```python
from build123d import *

# Parameters (mm, degrees)
SKETCH_1_R               = 32
EXTRUDE_1_DEPTH          = 10
EXTRUDE_2_DEPTH          = 10
PATTERN_CIRCULAR_1_COUNT = 3
SKETCH_3_R               = 23
EXTRUDE_3_DEPTH          = 28
SKETCH_4_R               = 15
CUT_EXTRUDE_1_DEPTH      = 88.68422222
SKETCH_5_R               = 19
CUT_EXTRUDE_2_DEPTH      = 9
SKETCH_6_R               = 4.5
CUT_EXTRUDE_3_DEPTH      = 84.836285858


with BuildPart() as part:
    # Sketch 1 → Extrude 1 (new body)
    with BuildSketch(Plane.XY):
        Circle(SKETCH_1_R)
    extrude(amount=EXTRUDE_1_DEPTH)

    # Sketch 2 → Extrude 2 (add)
    with BuildSketch(Plane.XY):
        with BuildLine():
            Line((20, -11), (48, -11))
            ThreePointArc((48, -11), (59, 0), (48, 11))
            Line((48, 11), (20, 11))
            ThreePointArc((20, 11), (9, 0), (20, -11))
        make_face()
    extrude_2 = extrude(amount=EXTRUDE_2_DEPTH)

    # Pattern Circular 1: Extrude 2 ×3 about axis
    pattern_circular_1_axis = Axis((0, 0, 0), (0, 0, 1))
    for i in range(1, PATTERN_CIRCULAR_1_COUNT):
        add(extrude_2.rotate(pattern_circular_1_axis, i * 360 / PATTERN_CIRCULAR_1_COUNT))

    # Sketch 3 → Extrude 3 (add)
    with BuildSketch(Plane.XY.offset(10)):
        Circle(SKETCH_3_R)
    extrude(amount=EXTRUDE_3_DEPTH)

    # Sketch 4 → Cut-Extrude 1 (cut, through all)
    with BuildSketch(Plane.XY.offset(38)):
        Circle(SKETCH_4_R)
    extrude(amount=-CUT_EXTRUDE_1_DEPTH, mode=Mode.SUBTRACT)

    # Sketch 5 → Cut-Extrude 2 (cut)
    with BuildSketch(Plane.XY.offset(38)):
        Circle(SKETCH_5_R)
    extrude(amount=-CUT_EXTRUDE_2_DEPTH, mode=Mode.SUBTRACT)

    # Sketch 6 → Cut-Extrude 3 (cut, through all)
    with BuildSketch(Plane.XY.offset(10)):
        with Locations((48, 0)):
            Circle(SKETCH_6_R)
        with Locations((-24, 41.569219)):
            Circle(SKETCH_6_R)
        with Locations((-24, -41.569219)):
            Circle(SKETCH_6_R)
    extrude(amount=-CUT_EXTRUDE_3_DEPTH, mode=Mode.SUBTRACT)


solid = part.part
```
Read the model definition and answer for the solid it produces. Units are mm, in the model's axes. A direction names the side the tool comes from. Give positions to 0.01 mm unless a question says otherwise; leave off trailing zeros. Order: outer loops, then holes, each group sorted by start corner. A loop starts at its lowest first (then second) coordinate and runs counter-clockwise, first axis right, second up. Notation, with made-up numbers: (65, 59) -> (99, 59) arc R13 cw to (99, 65) -> close; hole circle Ø7 at (58, 62.5). An arc over 180 degrees is marked (long way). Write item = value, one per line.
1. A cutting plane is placed at D-D, the plane y = -12.5. Write down the section's boundary in (x, z).
Numbers:
outline = (-29.46, 0) -> (-8.29, 0) -> (-8.29, 29) -> (-14.31, 29) -> (-14.31, 38) -> (-19.31, 38) -> (-19.31, 10) -> (-29.46, 10) -> close; (8.29, 0) -> (29.46, 0) -> (29.46, 10) -> (19.31, 10) -> (19.31, 38) -> (14.31, 38) -> (14.31, 29) -> (8.29, 29) -> close
2. Straight lines are drawn through the part: line 1 along X through (y, z) = (-3.5, 2.5); line 2 along Y through (x, z) = (0, 36); line 3 along Z through (x, y) = (-0.5, 15.5). For each, find the intervals that lie inside material, in ascending order.
Numbers:
line_1 = -31.81 to -14.59, 14.59 to 45.17, 50.83 to 58.43
line_2 = -23 to -19, 19 to 23
line_3 = 0 to 29
3. For faces 1 (the face through (-11, -21, 10)), 2 (the face through (-29.1, 28.4, 4.9)), 3 (the face through (39, -11, 5)), determine the directions among +Z, -Z, +X, -X, +Y, -Y from which every point of the face is accessible in a straight line to the end or side of a thin tool.
Numbers:
face_1 = +Z
face_2 = +Z, -Z, -X
face_3 = +Z, -Z, +X, -Y
4. Given pin 1 (2 mm diameter, centred on x = 3, z = 27.5, fed in from +Y); pin 2 (8 mm diameter, centred on x = 24, z = 25, fed in from -Y); pin 3 (11 mm diameter, centred on x = 41, z = 5.5, fed in from -Y), each flat-ended and moving along its own axis, determine where each tip first touches the part or whether it passes through.
Numbers:
pin_1 = 22.91
pin_2 = -11.36
pin_3 = -11
5. The mould has two halves that part along X. Classify faces 4 (the face through (14, 6, 29)), 5 (the face through (-2.994, 22.804, 23.804)), 6 (the face through (-28.976, -28.188, 4.93)): +X half, -X half, draft (parallel to the pull), parting line (faces both ways), or undercut.
Numbers:
face_4 = undercut
face_5 = parting line
face_6 = -X half
6. A cutting plane is placed at B-B, the plane y = 0. Write down the section's boundary in (x, z), and give its area (3 significant figures).
Numbers:
outline = (-32, 0) -> (-15, 0) -> (-15, 29) -> (-19, 29) -> (-19, 38) -> (-23, 38) -> (-23, 10) -> (-32, 10) -> close; (15, 0) -> (43.5, 0) -> (43.5, 10) -> (23, 10) -> (23, 38) -> (19, 38) -> (19, 29) -> (15, 29) -> close; (52.5, 0) -> (59, 0) -> (59, 10) -> (52.5, 10) -> close
area = 896 mm²
7. A cutting plane is placed at C-C, the plane z = 5. Write down the section's boundary in (x, y), and give its area (3 significant figures).
Numbers:
outline = (-33.53, -36.07) arc R11 ccw to (-14.47, -47.07) -> (-5.5, -31.52) arc R32 ccw to (30.05, -11) -> (48, -11) arc R11 ccw to (48, 11) -> (30.05, 11) arc R32 ccw to (-5.5, 31.52) -> (-14.47, 47.07) arc R11 ccw to (-33.53, 36.07) -> (-24.55, 20.52) arc R32 ccw to (-24.55, -20.52) -> close; hole circle Ø9 at (-24, -41.57); hole circle Ø9 at (-24, 41.57); hole circle Ø30 at (0, 0); hole circle Ø9 at (48, 0)
area = 3,990 mm²
8. A cutting plane is placed at A-A, the plane x = 0. Write down the section's boundary in (y, z).
Numbers:
outline = (-32, 0) -> (-15, 0) -> (-15, 29) -> (-19, 29) -> (-19, 38) -> (-23, 38) -> (-23, 10) -> (-32, 10) -> close; (15, 0) -> (32, 0) -> (32, 10) -> (23, 10) -> (23, 38) -> (19, 38) -> (19, 29) -> (15, 29) -> close
